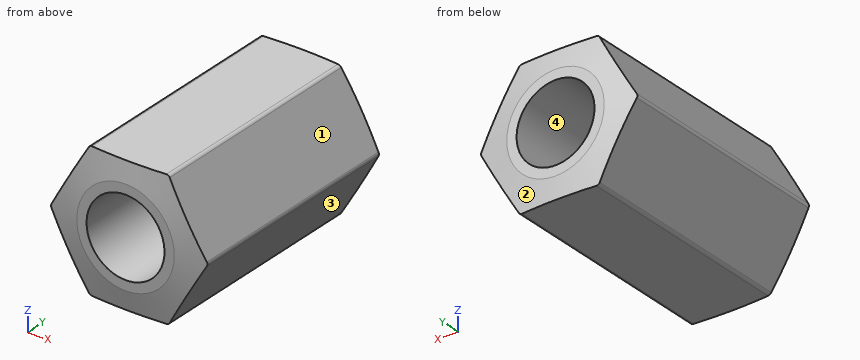
from build123d import *

# Parameters (mm, degrees)
EXTRUDE_1_DEPTH     = 6
FILLET_1_R          = 0.2
SKETCH_3_R          = 2
CUT_EXTRUDE_1_DEPTH = 8


with BuildPart() as part:
    # 草图1 → 凸台-拉伸1 (new, symmetric)
    with BuildSketch(Plane(origin=(0, 0, 0), x_dir=(1, 0, 0), z_dir=(0, 1, 0))):
        Polygon((4.041451884, 0), (2.020725942, 3.5), (-2.020725942, 3.5), (-4.041451884, 0), (-2.020725942, -3.5), (2.020725942, -3.5), align=None)
    extrude(amount=EXTRUDE_1_DEPTH, both=True)

    # 圆角1
    fillet_1_edges = [part.edges().sort_by_distance(p)[0] for p in [
        (2.020725942, 0, 3.5),
        (-2.020725942, 0, 3.5),
        (-4.041451884, 0, 0),
        (-2.020725942, 0, -3.5),
        (2.020725942, 0, -3.5),
        (4.041451884, 0, 0),
    ]]
    fillet(fillet_1_edges, radius=FILLET_1_R)

    # 草图3 → 切除-拉伸1 (cut)
    with BuildSketch(Plane(origin=(0, 6, 0), x_dir=(1, 0, 0), z_dir=(0, 1, 0))):
        with Locations(Location((0, 0, 0), (0, 0, 270))):
            Circle(SKETCH_3_R)
    cut_extrude_1 = extrude(amount=-CUT_EXTRUDE_1_DEPTH, mode=Mode.SUBTRACT)

    # 草图4 → 切除-旋转1 (revolve, cut)
    with BuildSketch(Plane.XY, mode=Mode.PRIVATE) as cut_revolve_1_sk:
        Polygon((-4.010511777, 6), (-4.010511777, 5.75), (-2.5, 6), align=None)
    cut_revolve_1 = revolve(cut_revolve_1_sk.sketch.rotate(Axis((0, 0, 0), (0, 1, 0)), 180), axis=Axis((0, 0, 0), (0, 1, 0)), mode=Mode.SUBTRACT)

    # 镜向1: 切除-拉伸1, 切除-旋转1 across plane
    add(cut_extrude_1.mirror(Plane.ZX), mode=Mode.SUBTRACT)
    add(cut_revolve_1.mirror(Plane.ZX), mode=Mode.SUBTRACT)


solid = part.part
The model under review builds one solid part; all positions refer to its coordinate system, in mm. Face numbers are marked on the shaded views. Coordinates: 2 decimals unless noted, no trailing zeros. Loops run counter-clockwise (first coordinate to the right, second up) from the corner with the lowest first, then second, coordinate; pieces in that order, holes last.
(1) Consider section A-A, the plane x = 0. Give the boundary of the cut face in (y, z), plus the area to 3 significant figures.
Determined:
outline: (-6, -2.5) - (-5.83, -3.5) - (5.83, -3.5) - (6, -2.5) - (6, -2) - (-6, -2) - close; (-6, 2) - (6, 2) - (6, 2.5) - (5.83, 3.5) - (-5.83, 3.5) - (-6, 2.5) - close
area: 35.7 mm2
(2) Wall thickness on L1, parallel to X at y = 0.5, z = -1; L2, parallel to X at y = -2.75, z = -0.25; L3, parallel to Z at x = 1.5, y = -1: over which ranges is each line inside the solid? List them lowest first.
Determined:
L1: x = -3.46 to -1.73, 1.73 to 3.46
L2: x = -3.9 to -1.98, 1.98 to 3.9
L3: z = -3.5 to -1.32, 1.32 to 3.5
(3) Consider section B-B, the plane y = 4.25. Give the boundary of the cut face in (x, z), plus the area to 3 significant figures.
Determined:
outline: (-3.98, -0.1) - (-2.08, -3.4) arc R0.2 ccw to (-1.91, -3.5) - (1.91, -3.5) arc R0.2 ccw to (2.08, -3.4) - (3.98, -0.1) arc R0.2 ccw to (3.98, 0.1) - (2.08, 3.4) arc R0.2 ccw to (1.91, 3.5) - (-1.91, 3.5) arc R0.2 ccw to (-2.08, 3.4) - (-3.98, 0.1) arc R0.2 ccw to start; hole circle Ø4 at (0, 0)
area: 29.9 mm2
(4) Insertion check: P1, Ø3.5, axis at x = 0, z = 0, coming from the -Y side. The pin has a flat end and moves straight along its axis. Give the tip position at first contact, or say it passes through.
Determined:
P1: passes through
(5) Draft analysis for pull direction Z (two halves, no side actions). For the marked faces 1, 2, 3 and 4, state which applies: +Z half, -Z half, draft (parallel to the pull), parting line (faces both ways), or undercut.
Determined:
face 1: +Z half
face 2: parting line
face 3: -Z half
face 4: undercut
